from build123d import *

# Parameters (mm, degrees)
DODANIE_WYCI_GNI_CIE1_DEPTH = 27.5
SZKIC2_W                    = 111
SZKIC2_H                    = 21.5
WYTNIJ_WYCI_GNI_CIE1_DEPTH  = 30.5
SZKIC3_W                    = 20
SZKIC3_H                    = 15
WYTNIJ_WYCI_GNI_CIE2_DEPTH  = 3
SZKIC4_W                    = 20.5
SZKIC4_H                    = 20
WYTNIJ_WYCI_GNI_CIE3_DEPTH  = 3
SZKIC5_R                    = 1.6
WYTNIJ_WYCI_GNI_CIE4_DEPTH  = 133.064614867


with BuildPart() as part:
    # Szkic1 → Dodanie-wyciągnięcie1 (new body)
    with BuildSketch(Plane.XY):
        Polygon((0, 0), (117, 0), (117, 28.5), (124.75, 28.5), (124.75, 33.5), (-7.75, 33.5), (-7.75, 28.5), (0, 28.5), align=None)
    extrude(amount=DODANIE_WYCI_GNI_CIE1_DEPTH)

    # Szkic2 → Wytnij-wyciągnięcie1 (cut)
    with BuildSketch(Plane(origin=(0, 33.5, 0), x_dir=(1, 0, 0), z_dir=(0, 1, 0))):
        with Locations((58.5, -13.75)):
            Rectangle(SZKIC2_W, SZKIC2_H)
    extrude(amount=-WYTNIJ_WYCI_GNI_CIE1_DEPTH, mode=Mode.SUBTRACT)

    # Szkic3 → Wytnij-wyciągnięcie2 (cut)
    with BuildSketch(Plane(origin=(117, 0, 0), x_dir=(0, 0, -1), z_dir=(1, 0, 0))):
        with Locations((-13.9, 18.5)):
            Rectangle(SZKIC3_W, SZKIC3_H)
    extrude(amount=-WYTNIJ_WYCI_GNI_CIE2_DEPTH, mode=Mode.SUBTRACT)

    # Szkic4 → Wytnij-wyciągnięcie3 (cut)
    with BuildSketch(Plane.ZY):
        with Locations((13.75, 18.5)):
            Rectangle(SZKIC4_W, SZKIC4_H)
    extrude(amount=-WYTNIJ_WYCI_GNI_CIE3_DEPTH, mode=Mode.SUBTRACT)

    # Szkic5 → Wytnij-wyciągnięcie4 (cut, through all)
    with BuildSketch(Plane(origin=(0, 33.5, 0), x_dir=(1, 0, 0), z_dir=(0, 1, 0))):
        with Locations(Location((-3.75, -4, 0), (0, 0, 180))):
            Circle(SZKIC5_R)
        with Locations(Location((120.75, -4, 0), (0, 0, 180))):
            Circle(SZKIC5_R)
        with Locations(Location((120.75, -24, 0), (0, 0, 180))):
            Circle(SZKIC5_R)
        with Locations(Location((-3.75, -24, 0), (0, 0, 180))):
            Circle(SZKIC5_R)
    extrude(amount=-WYTNIJ_WYCI_GNI_CIE4_DEPTH, mode=Mode.SUBTRACT)


solid = part.part
Could you check a few things on this model? Use its own coordinates, in mm. A direction names the side the tool comes from. Round coordinates to 2 decimals unless told otherwise and drop trailing zeros. Order: outer loops, then holes, each group sorted by start corner. A loop starts at its lowest first (then second) coordinate and runs counter-clockwise, first axis right, second up.
(1) Imagine slicing it at A-A (z = 14.5). Write out the boundary of the cut face in (x, y).
Response values:
outline: (-7.75, 28.5) - (3, 28.5) - (3, 33.5) - (-7.75, 33.5) - close; (0, 0) - (117, 0) - (117, 11) - (114, 11) - (114, 3) - (3, 3) - (3, 8.5) - (0, 8.5) - close; (114, 26) - (117, 26) - (117, 28.5) - (124.75, 28.5) - (124.75, 33.5) - (114, 33.5) - close
(2) Imagine slicing it at D-D (x = 100). Write out the boundary of the cut face in (y, z).
Response values:
outline: (0, 0) - (33.5, 0) - (33.5, 3) - (3, 3) - (3, 24.5) - (33.5, 24.5) - (33.5, 27.5) - (0, 27.5) - close
(3) Please list where these lines run through material, in increasing order: line 1 along Z through (x, y) = (-3.75, 30.75); line 2 along X through (y, z) = (5, 19.5); line 3 along Z through (x, y) = (32.5, 4).
Response values:
line 1: z = 0 to 2.4, 5.6 to 22.4, 25.6 to 27.5
line 2: x = 0 to 3, 114 to 117
line 3: z = 0 to 3, 24.5 to 27.5
(4) I'm going to push flat-ended pins straight in: pin 1 (3 mm diameter, centred on y = 22.5, z = 3, fed in from -X); pin 2 (11 mm diameter, centred on y = 18.5, z = 18.5, fed in from +X); pin 3 (6.5 mm diameter, centred on x = 77.5, z = 18, fed in from +Y). Where does each tip first touch, or does it pass through?
Response values:
pin 1: stops at x = 0
pin 2: stops at x = 117
pin 3: stops at y = 3
(5) Which directions (+Z, -Z, +X, -X, +Y, -Y) give clear straight access to the entire face, cutting with the end or side of a thin tool? Please do faces 5 (the flat face through (116, 18, 3.9)), 6 (the flat face through (121, 28.5, 14)), 7 (the flat face through (1, 18, 24)), 8 (the flat face through (114, 8, 14)), 9 (the flat face through (0, 8, 14)).
Response values:
face 5: +X, -X
face 6: +Z, -Z, +X, -Y
face 7: -X
face 8: +Y
face 9: +Z, -Z, -X, -Y
(6) Imagine slicing it at B-B (x = 120.75). Write out the boundary of the cut face in (y, z).
Response values:
outline: (28.5, 0) - (33.5, 0) - (33.5, 2.4) - (28.5, 2.4) - close; (28.5, 5.6) - (33.5, 5.6) - (33.5, 22.4) - (28.5, 22.4) - close; (28.5, 25.6) - (33.5, 25.6) - (33.5, 27.5) - (28.5, 27.5) - close
(7) If we mould it in two halves opening along Z, with no side actions, what happens to faces 1 (the cylindrical face through (119.224, 31.035, 24.481)), 2 (the flat face through (-7.75, 31, 14)), 3 (the flat face through (58, 17, 27.5)), 4 (the flat face through (58, 3, 14))? For each: released by +Z, released by -Z, zero draft, split by the parting line, or undercut.
Response values:
face 1: undercut
face 2: zero draft
face 3: released by +Z
face 4: undercut
(8) Imagine slicing it at C-C (y = 23). Write out the boundary of the cut face in (x, z), plus the area to 4 significant figures.
Response values:
outline: (0, 0) - (117, 0) - (117, 3.9) - (114, 3.9) - (114, 3) - (3, 3) - (3, 3.5) - (0, 3.5) - close; (0, 24) - (3, 24) - (3, 24.5) - (114, 24.5) - (114, 23.9) - (117, 23.9) - (117, 27.5) - (0, 27.5) - close
area: 709.5 mm2
